Model file for the job. Use its own axes, mm. Face numbers are marked on the shaded views. Coordinates: 2 decimals unless noted, no trailing zeros. Order: outer loops, then holes, each group sorted by start corner. A loop starts at its lowest first (then second) coordinate and runs counter-clockwise, first axis right, second up. Notation, with made-up numbers: M 68,30.25 L 109,30.25 A4 cw 109,34.25 Z; hole C 83.5,42.25 d5. An arc over 180 degrees is marked long. Return JSON: item names as keys, results as strings.
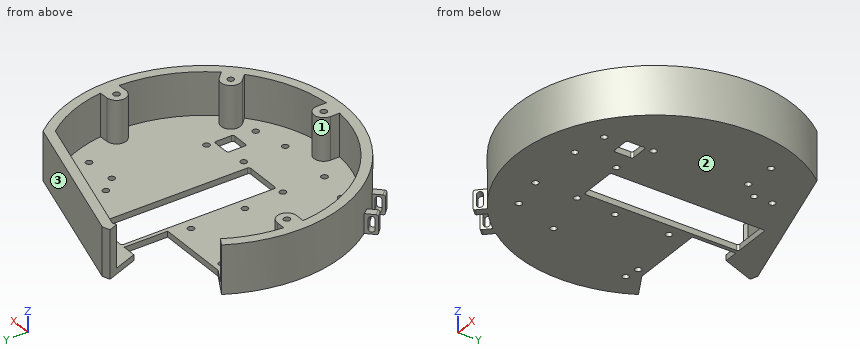
```python
from build123d import *

# Parameters (mm, degrees)
SKETCH1_R                 = 71.545
SKETCH1_R_2               = 1.65
PLATE_EXTRUD_DEPTH        = 3
SKETCH2_R                 = 1.65
ARDUINO_MOUNT_HOLES_DEPTH = 3
CABLE_HOLE_DEPTH          = 102.224374782
SKETCH5_R                 = 1.65
RELAY_MOUNT_HOLES_DEPTH   = 102.224374782
SKETCH6_R                 = 1.65
BOSS_EXTRUDE3_DEPTH       = 25
CUT_EXTRUDE1_DEPTH        = 105.222713695
CUT_EXTRUDE2_START        = 22
CUT_EXTRUDE2_DEPTH        = 2.6
CUT_EXTRUDE3_DEPTH        = 105.222713695
BOSS_EXTRUDE4_DEPTH       = 10
BOSS_EXTRUDE4_DEPTH_BACK  = 10
CUT_EXTRUDE4_DEPTH        = 105.222713695
SKETCH12_R                = 1.65
CUT_EXTRUDE5_DEPTH        = 105.222713695


with BuildPart() as part:
    # Sketch1 → Plate extrud (new body)
    with BuildSketch(Plane(origin=(0, 0, 0), x_dir=(0, 1, 0), z_dir=(0, 0, 1))):
        with Locations(Location((0, 0, 0), (0, 0, 270))):
            Circle(SKETCH1_R)
        with Locations(Location((-48.5, 32, 0), (0, 0, 270))):
            Circle(SKETCH1_R_2, mode=Mode.SUBTRACT)
        with Locations(Location((22, 54, 0), (0, 0, 270))):
            Circle(SKETCH1_R_2, mode=Mode.SUBTRACT)
        with Locations(Location((24, -52, 0), (0, 0, 270))):
            Circle(SKETCH1_R_2, mode=Mode.SUBTRACT)
        with Locations(Location((-48.5, -32, 0), (0, 0, 270))):
            Circle(SKETCH1_R_2, mode=Mode.SUBTRACT)
    extrude(amount=PLATE_EXTRUD_DEPTH)

    # Sketch2 → Arduino mount holes (cut)
    with BuildSketch(Plane(origin=(0, 0, 0), x_dir=(0, 1, 0), z_dir=(0, 0, 1))):
        with Locations(Location((-25, 40, 0), (0, 0, 270))):
            Circle(SKETCH2_R)
        with Locations(Location((23.22, 46.36, 0), (0, 0, 270))):
            Circle(SKETCH2_R)
        with Locations(Location((18.14, 15.91, 0), (0, 0, 270))):
            Circle(SKETCH2_R)
        with Locations(Location((-9.77, 15.91, 0), (0, 0, 270))):
            Circle(SKETCH2_R)
        with Locations(Location((-25, -34.88, 0), (0, 0, 270))):
            Circle(SKETCH2_R)
        with Locations(Location((23.22, -36.11, 0), (0, 0, 270))):
            Circle(SKETCH2_R)
    extrude(amount=ARDUINO_MOUNT_HOLES_DEPTH, mode=Mode.SUBTRACT)

    # Sketch4 → Cable hole (cut, through all)
    with BuildSketch(Plane(origin=(0, 0, 0), x_dir=(0, 1, 0), z_dir=(0, 0, 1))):
        with BuildLine():
            Line((-29, 10), (49, 10))
            ThreePointArc((49, 10), (49.707106781, 9.707106781), (50, 9))
            Line((50, 9), (50, -9))
            ThreePointArc((50, -9), (49.707106781, -9.707106781), (49, -10))
            Line((49, -10), (-29, -10))
            ThreePointArc((-29, -10), (-29.707106781, -9.707106781), (-30, -9))
            Line((-30, -9), (-30, 9))
            ThreePointArc((-30, 9), (-29.707106781, 9.707106781), (-29, 10))
        make_face()
        with BuildLine():
            Line((-38, -25), (-30, -25))
            ThreePointArc((-30, -25), (-29.292893219, -25.292893219), (-29, -26))
            Line((-29, -26), (-29, -34))
            ThreePointArc((-29, -34), (-29.292893219, -34.707106781), (-30, -35))
            Line((-30, -35), (-38, -35))
            ThreePointArc((-38, -35), (-38.707106781, -34.707106781), (-39, -34))
            Line((-39, -34), (-39, -26))
            ThreePointArc((-39, -26), (-38.707106781, -25.292893219), (-38, -25))
        make_face()
    extrude(amount=CABLE_HOLE_DEPTH, mode=Mode.SUBTRACT)

    # Sketch5 → Relay mount holes (cut, through all)
    with BuildSketch(Plane(origin=(0, 0, 0), x_dir=(0, 1, 0), z_dir=(0, 0, 1))):
        with Locations(Location((-52, -15, 0), (0, 0, 270))):
            Circle(SKETCH5_R)
        with Locations(Location((-30.5, -15, 0), (0, 0, 270))):
            Circle(SKETCH5_R)
        with Locations(Location((-30.5, 14.4, 0), (0, 0, 270))):
            Circle(SKETCH5_R)
        with Locations(Location((-52, 14.4, 0), (0, 0, 270))):
            Circle(SKETCH5_R)
    extrude(amount=RELAY_MOUNT_HOLES_DEPTH, mode=Mode.SUBTRACT)

    # Sketch6 → Boss-Extrude3 (add)
    with BuildSketch(Plane(origin=(0, 0, 0), x_dir=(0, 1, 0), z_dir=(0, 0, 1))):
        with BuildLine():
            ThreePointArc((68.149505263, 21.779163377), (-68.679774221, 20.044341793), (45.736375855, -55.017005995))
            Line((45.736375855, -55.017005995), (68.149505263, 21.779163377))
        make_face()
        with BuildLine():
            ThreePointArc((-66.356891315, -5), (-66.545, 0), (-66.356891315, 5))
            ThreePointArc((-66.356891315, 5), (-47.054420754, 47.054420754), (-5, 66.356891315))
            Line((-5, 66.356891315), (-5, 61.545))
            ThreePointArc((-5, 61.545), (0, 56.545), (5, 61.545))
            Line((5, 61.545), (5, 66.356891315))
            ThreePointArc((5, 66.356891315), (40.644418881, 52.69030498), (62.91305896, 21.683727477))
            Line((62.91305896, 21.683727477), (41.373300987, -52.119928918))
            ThreePointArc((41.373300987, -52.119928918), (25.868565875, -61.311127249), (8.465999034, -66.004271721))
            ThreePointArc((8.465999034, -66.004271721), (3.482696208, -66.45380239), (-1.520296313, -66.527631283))
            ThreePointArc((-1.520296313, -66.527631283), (-23.847595202, -62.125109481), (-43.385873921, -50.456941733))
            ThreePointArc((-43.385873921, -50.456941733), (-47.054420754, -47.054420754), (-50.456941733, -43.385873921))
            ThreePointArc((-50.456941733, -43.385873921), (-61.479563491, -25.465669007), (-66.356891315, -5))
        make_face(mode=Mode.SUBTRACT)
        with Locations(Location((0, 61.545, 0), (0, 0, 270))):
            Circle(SKETCH6_R, mode=Mode.SUBTRACT)
        with BuildLine():
            ThreePointArc((68.149505263, 21.779163377), (-68.679774221, 20.044341793), (45.736375855, -55.017005995))
            Line((45.736375855, -55.017005995), (68.149505263, 21.779163377))
        make_face()
        with BuildLine():
            ThreePointArc((-66.356891315, -5), (-66.545, 0), (-66.356891315, 5))
            ThreePointArc((-66.356891315, 5), (-47.054420754, 47.054420754), (-5, 66.356891315))
            Line((-5, 66.356891315), (-5, 61.545))
            ThreePointArc((-5, 61.545), (0, 56.545), (5, 61.545))
            Line((5, 61.545), (5, 66.356891315))
            ThreePointArc((5, 66.356891315), (40.644418881, 52.69030498), (62.91305896, 21.683727477))
            Line((62.91305896, 21.683727477), (41.373300987, -52.119928918))
            ThreePointArc((41.373300987, -52.119928918), (25.868565875, -61.311127249), (8.465999034, -66.004271721))
            ThreePointArc((8.465999034, -66.004271721), (3.482696208, -66.45380239), (-1.520296313, -66.527631283))
            ThreePointArc((-1.520296313, -66.527631283), (-23.847595202, -62.125109481), (-43.385873921, -50.456941733))
            ThreePointArc((-43.385873921, -50.456941733), (-47.054420754, -47.054420754), (-50.456941733, -43.385873921))
            ThreePointArc((-50.456941733, -43.385873921), (-61.479563491, -25.465669007), (-66.356891315, -5))
        make_face(mode=Mode.SUBTRACT)
        with Locations(Location((0, 61.545, 0), (0, 0, 270))):
            Circle(SKETCH6_R, mode=Mode.SUBTRACT)
        with BuildLine():
            ThreePointArc((-66.356891315, -5), (-66.545, 0), (-66.356891315, 5))
            Line((-66.356891315, 5), (-61.545, 5))
            ThreePointArc((-61.545, 5), (-56.545, 0), (-61.545, -5))
            Line((-61.545, -5), (-66.356891315, -5))
        make_face()
        with Locations(Location((-61.545, 0, 0), (0, 0, 270))):
            Circle(SKETCH6_R, mode=Mode.SUBTRACT)
        with BuildLine():
            Line((-1.772131247, -61.722334498), (-1.520296313, -66.527631283))
            ThreePointArc((-1.520296313, -66.527631283), (3.482696208, -66.45380239), (8.465999034, -66.004271721))
            Line((8.465999034, -66.004271721), (8.214164101, -61.198974935))
            ThreePointArc((8.214164101, -61.198974935), (2.959336646, -56.467507043), (-1.772131247, -61.722334498))
        make_face()
        with Locations(Location((3.221016427, -61.460654716, 0), (0, 0, 270))):
            Circle(SKETCH6_R, mode=Mode.SUBTRACT)
        with BuildLine():
            Line((-47.054420754, -39.983352942), (-50.456941733, -43.385873921))
            ThreePointArc((-50.456941733, -43.385873921), (-47.054420754, -47.054420754), (-43.385873921, -50.456941733))
            Line((-43.385873921, -50.456941733), (-39.983352942, -47.054420754))
            ThreePointArc((-39.983352942, -47.054420754), (-39.983352942, -39.983352942), (-47.054420754, -39.983352942))
        make_face()
        with Locations(Location((-43.518886848, -43.518886848, 0), (0, 0, 270))):
            Circle(SKETCH6_R, mode=Mode.SUBTRACT)
    extrude(amount=BOSS_EXTRUDE3_DEPTH)

    # Sketch7 → Cut-Extrude1 (cut, through all)
    with BuildSketch(Plane.XY.offset(25)):
        with BuildLine():
            Line((-21.779163377, 68.149505263), (55.017005995, 45.736375855))
            ThreePointArc((55.017005995, 45.736375855), (20.044341793, 68.679774221), (-21.779163377, 68.149505263))
        make_face()
    extrude(amount=-CUT_EXTRUDE1_DEPTH, mode=Mode.SUBTRACT)

    # Sketch8 → Cut-Extrude2 (cut)
    with BuildSketch(Plane(origin=(0, 0, 0), x_dir=(0, 1, 0), z_dir=(0, 0, 1)).offset(CUT_EXTRUDE2_START)):
        Polygon((-60.154258671, 2.854675444), (-63.321850789, 2.631755043), (-64.712592118, -0.2229204), (-62.935741329, -2.854675444), (-59.768149211, -2.631755043), (-58.377407882, 0.2229204), align=None)
        Polygon((2.962348959, 60.401399554), (2.471561517, 63.53866923), (-0.490787442, 64.682269676), (-2.962348959, 62.688600446), (-2.471561517, 59.55133077), (0.490787442, 58.407730324), align=None)
        Polygon((6.396442908, -61.460654716), (4.808729667, -58.710654716), (1.633303187, -58.710654716), (0.045589946, -61.460654716), (1.633303187, -64.210654716), (4.808729667, -64.210654716), align=None)
        Polygon((-40.343460368, -43.518886848), (-41.931173608, -40.768886848), (-45.106600088, -40.768886848), (-46.694313329, -43.518886848), (-45.106600088, -46.268886848), (-41.931173608, -46.268886848), align=None)
    extrude(amount=-CUT_EXTRUDE2_DEPTH, mode=Mode.SUBTRACT)

    # Sketch9 → Cut-Extrude3 (cut, through all)
    with BuildSketch(Plane(origin=(0, 0, 0), x_dir=(0, 1, 0), z_dir=(0, 0, 1))):
        with BuildLine():
            Line((66.793011614, 25.63943495), (50, 19.193201752))
            Line((50, 19.193201752), (50, 12))
            Line((50, 12), (27.5, 12))
            Line((27.5, 12), (27.5, 49.795620732))
            Line((27.5, 49.795620732), (34.587369472, 62.629073903))
            ThreePointArc((34.587369472, 62.629073903), (53.95881545, 46.980136869), (66.793011614, 25.63943495))
        make_face()
    extrude(amount=CUT_EXTRUDE3_DEPTH, mode=Mode.SUBTRACT)

    # Sketch10 → Boss-Extrude4 (add, two sides)
    with BuildSketch(Plane(origin=(0, 0, 0), x_dir=(0.7071067811865477, 0.7071067811865475, 0), z_dir=(-0.7071067811865475, 0.7071067811865477, 0))) as boss_extrude4_sk:
        with BuildLine():
            Line((-67.545, 0), (-76.045, 0))
            ThreePointArc((-76.045, 0), (-76.752106781, -0.292893219), (-77.045, -1))
            Line((-77.045, -1), (-77.045, -9))
            ThreePointArc((-77.045, -9), (-76.752106781, -9.707106781), (-76.045, -10))
            Line((-76.045, -10), (-67.545, -10))
            Line((-67.545, -10), (-67.545, 0))
        make_face()
        with BuildLine():
            Line((-72.545, -2.5), (-72.545, -7.5))
            ThreePointArc((-72.545, -7.5), (-74.045, -9), (-75.545, -7.5))
            Line((-75.545, -7.5), (-75.545, -2.5))
            ThreePointArc((-75.545, -2.5), (-74.045, -1), (-72.545, -2.5))
        make_face(mode=Mode.SUBTRACT)
    extrude(amount=BOSS_EXTRUDE4_DEPTH)
    extrude(boss_extrude4_sk.sketch, amount=-BOSS_EXTRUDE4_DEPTH_BACK)

    # Sketch11 → Cut-Extrude4 (cut, through all)
    with BuildSketch(Plane(origin=(0, 0, 0), x_dir=(0, 1, 0), z_dir=(0, 0, 1))):
        with BuildLine():
            Line((-54.654380515, 46.169099141), (-58.721682644, 50.236401269))
            Line((-58.721682644, 50.236401269), (-50.236401269, 58.721682644))
            Line((-50.236401269, 58.721682644), (-46.169099141, 54.654380515))
            ThreePointArc((-46.169099141, 54.654380515), (-50.58995466, 50.58995466), (-54.654380515, 46.169099141))
        make_face()
    extrude(amount=CUT_EXTRUDE4_DEPTH, mode=Mode.SUBTRACT)

    # Sketch12 → Cut-Extrude5 (cut, through all)
    with BuildSketch(Plane(origin=(0, 0, 0), x_dir=(0, 1, 0), z_dir=(0, 0, 1))):
        with Locations(Location((30.82, -29.5, 0), (0, 0, 270))):
            Circle(SKETCH12_R)
        with Locations(Location((40.18, -29.5, 0), (0, 0, 270))):
            Circle(SKETCH12_R)
    extrude(amount=CUT_EXTRUDE5_DEPTH, mode=Mode.SUBTRACT)


solid = part.part
```
Item 1: Drop flat-ended pins along their axis: pin 1 Ø2 at (x, z) = (29, 12) entering from +Y; pin 2 Ø2.5 at (x, y) = (-61.5, 0) entering from +Z; pin 3 Ø0.9 at (x, z) = (-1.5, 1) entering from +Y. Give the stop position or say it passes through.
Check result:
{"pin 1": "stops at y = 53.62", "pin 2": "stops at z = 3", "pin 3": "stops at y = 62.36"}
Item 2: Pull direction Y, two halves, no side cores. Call the marked faces 1, 2 and 3: +Y half, -Y half, draft (parallel to the pull), parting line (faces both ways), or undercut.
Check result:
{"face 1": "undercut", "face 2": "draft", "face 3": "+Y half"}
Item 3: Saw through at C-C (y = 53.5). Write the cut outline in (x, z), and give its area (3 significant figures).
Check result:
{"outline": "M -20.54,0 L 28.42,0 L 28.42,25 L 10.57,25 L 10.57,3 L -20.54,3 Z", "area": "539 mm2"}
Item 4: Saw through at B-B (z = 16). Count the separate pieces of the cut face and the enclosed holes in it, and give its area (3 significant figures).
Check result:
{"separate pieces": "1", "enclosed holes": "4", "area": "2,220 mm2"}
Item 5: Wall check: line 1 (X direction, y = -43, z = 14); line 2 (X direction, y = -44.5, z = 11); line 3 (X direction, y = 2, z = 4). Give the ranges that are in metal, low to high.
Check result:
{"line 1": "x = -57.18 to -50.79, 38.55 to 41.95, 45.09 to 50.07, 50.79 to 57.18", "line 2": "x = -56.02 to -49.48, 38.62 to 42.19, 44.85 to 56.02", "line 3": "x = -71.52 to -56.96, 56.61 to 60.35, 62.57 to 71.52"}
Item 6: Saw through at A-A (x = 20). Write the cut outline in (y, z), and give its area (3 significant figures).
Check result:
{"outline": "M -68.69,0 L 55.96,0 L 55.96,25 L 50.75,25 L 50.75,3 L -63.47,3 L -63.47,25 L -68.69,25 Z", "area": "603 mm2"}
